Work out the finished part from the listing and answer in its coordinate system (mm). Face numbers are marked on the shaded views. A direction names the side the tool comes from. Round coordinates to 2 decimals unless told otherwise and drop trailing zeros. Order: outer loops, then holes, each group sorted by start corner. A loop starts at its lowest first (then second) coordinate and runs counter-clockwise, first axis right, second up. Notation, with made-up numbers: (79, 62.5) - (133, 62.5) arc R19 cw to (133, 98.5) - close; hole circle Ø3 at (50, 49). An arc over 180 degrees is marked (long way). One line per question, with ' | ' between items. Start each with the question number.
from build123d import *

# Parameters (mm, degrees)
SKETCH1_W           = 40
SKETCH1_H           = 100
BOSS_EXTRUDE1_DEPTH = 8
SKETCH2_W           = 100
SKETCH2_H           = 53
BOSS_EXTRUDE2_DEPTH = 8
SKETCH3_R           = 2.65
CUT_EXTRUDE1_DEPTH  = 9
FILLET1_R           = 6
CHAMFER2_SIZE       = 10
FILLET3_R           = 9
CUT_EXTRUDE3_DEPTH  = 9
CHAMFER1_SIZE       = 5


with BuildPart() as part:
    # Sketch1 → Boss-Extrude1 (new body)
    with BuildSketch(Plane(origin=(0, 0, 0), x_dir=(1, 0, 0), z_dir=(0, 1, 0))):
        with Locations((20, 50)):
            Rectangle(SKETCH1_W, SKETCH1_H)
    extrude(amount=BOSS_EXTRUDE1_DEPTH)

    # Sketch2 → Boss-Extrude2 (add)
    with BuildSketch(Plane.ZY):
        with Locations((-50, 26.5)):
            Rectangle(SKETCH2_W, SKETCH2_H)
    extrude(amount=-BOSS_EXTRUDE2_DEPTH)

    # Sketch3 → Cut-Extrude1 (cut, through all)
    with BuildSketch(Plane(origin=(8, 0, 0), x_dir=(0, 0, -1), z_dir=(1, 0, 0))):
        with Locations((7.5, 48)):
            Circle(SKETCH3_R)
        with Locations((92.5, 28)):
            Circle(SKETCH3_R)
        with Locations((92.5, 48)):
            Circle(SKETCH3_R)
        with Locations((92.5, 38)):
            Circle(SKETCH3_R)
        with Locations((7.5, 28)):
            Circle(SKETCH3_R)
        with Locations((7.5, 38)):
            Circle(SKETCH3_R)
    extrude(amount=-CUT_EXTRUDE1_DEPTH, mode=Mode.SUBTRACT)

    # Fillet1
    fillet1_edges = [part.edges().sort_by_distance(p)[0] for p in [
        (4, 53, 0),
        (4, 53, -100),
    ]]
    fillet(fillet1_edges, radius=FILLET1_R)

    # Chamfer2
    chamfer2_edges = [part.edges().sort_by_distance(p)[0] for p in [
        (8, 8, -50),
    ]]
    chamfer(chamfer2_edges, length=CHAMFER2_SIZE)

    # Fillet3
    fillet3_edges = [part.edges().sort_by_distance(p)[0] for p in [
        (40, 4, -100),
        (40, 4, 0),
    ]]
    fillet(fillet3_edges, radius=FILLET3_R)

    # Sketch5 → Cut-Extrude3 (cut, through all)
    with BuildSketch(Plane(origin=(0, 8, 0), x_dir=(1, 0, 0), z_dir=(0, 1, 0))):
        with BuildLine():
            Line((33.65, 91), (33.65, 66))
            ThreePointArc((33.65, 66), (31, 63.35), (28.35, 66))
            Line((28.35, 66), (28.35, 91))
            ThreePointArc((28.35, 91), (31, 93.65), (33.65, 91))
        make_face()
        with BuildLine():
            Line((33.65, 34), (33.65, 9))
            ThreePointArc((33.65, 9), (31, 6.35), (28.35, 9))
            Line((28.35, 9), (28.35, 34))
            ThreePointArc((28.35, 34), (31, 36.65), (33.65, 34))
        make_face()
    extrude(amount=-CUT_EXTRUDE3_DEPTH, mode=Mode.SUBTRACT)

    # Chamfer1
    chamfer1_edges = [part.edges().sort_by_distance(p)[0] for p in [
        (0, 0, -50),
    ]]
    chamfer(chamfer1_edges, length=CHAMFER1_SIZE)


with BuildPart() as body_2:
    # Mirror1: mirrored copy
    add(part.part.mirror(Plane(origin=(0, 8, 0), x_dir=(0, 0, 1), z_dir=(1, 0, 0))))


solid = body_2.part
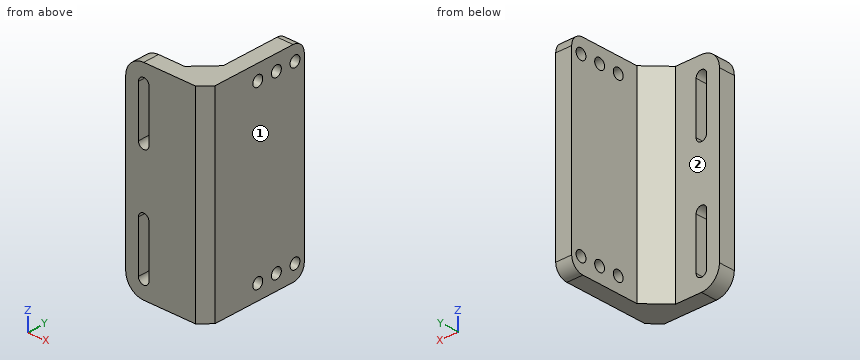
1) Straight lines are drawn through the part: line 1 (Y direction, x = -30.5, z = -47); line 2 (Y direction, x = -2, z = -7); line 3 (Y direction, x = -3, z = -7.5). For each, find the intervals that lie inside material, in ascending order.
2) For the marked faces 1 and 2, determine the directions among +Z, -Z, +X, -X, +Y, -Y from which every point of the face is accessible in a straight line to the end or side of a thin tool.
3) Section C-C on z = -39 is taken. Give the vertices of the cut face in (x, y).
4) Flat-ended cylindrical pins translate along their axes: pin 1 (3 mm diameter, centred on x = -23.5, z = -48.5, fed in from +Y); pin 2 (2.5 mm diameter, centred on y = 2.5, z = -74.5, fed in from +X); pin 3 (5 mm diameter, centred on x = -13.5, z = -73, fed in from +Y). Find the tip coordinate at first contact, or state that the pin passes through.
5) Section A-A on z = -75 is taken. Give the vertices of the cut face in (x, y).
6) Section B-B on y = 38 is taken. Give the vertices of the cut face in (x, z).
7) Section D-D on x = -21.5 is taken. Give the vertices of the cut face in (y, z), and give its area (3 significant figures).
Recorded:
1) line 1: y = 0 to 8 | line 2: y = 3 to 25.4, 30.6 to 35.4, 40.6 to 45.4, 50.6 to 53 | line 3: y = 2 to 25.35, 30.65 to 35.35, 40.65 to 45.35, 50.65 to 53
2) face 1: +Z, -Z, +X, +Y, -Y | face 2: +Z, -Z, -X, +Y
3) outline: (-40, 0) - (-5, 0) - (0, 5) - (0, 53) - (-8, 53) - (-8, 18) - (-18, 8) - (-40, 8) - close
4) pin 1: stops at y = 8 | pin 2: stops at x = -1.25 | pin 3: stops at y = 15
5) outline: (-40, 0) - (-33.65, 0) - (-33.65, 8) - (-40, 8) - close; (-28.35, 0) - (-5, 0) - (0, 5) - (0, 53) - (-8, 53) - (-8, 18) - (-18, 8) - (-28.35, 8) - close
6) outline: (-8, -100) - (0, -100) - (0, -95.15) - (-8, -95.15) - close; (-8, -89.85) - (0, -89.85) - (0, -10.15) - (-8, -10.15) - close; (-8, -4.85) - (0, -4.85) - (0, 0) - (-8, 0) - close
7) outline: (0, -100) - (8, -100) - (8, 0) - (0, 0) - close | area: 800 mm²
